Answer from the drawing. Dimensions are ordinates in mm from the lowest x, y and z of the part. A direction names the side the tool comes from. Give positions to 0.01 mm unless a question says otherwise; leave off trailing zeros. Loops run counter-clockwise (first coordinate to the right, second up) from the corner with the lowest first, then second, coordinate; pieces in that order, holes last.
Item 1: Consider line 1 along X through (y, z) = (29, 45) (1 decimal); line 2 along Y through (x, z) = (159, 42); line 3 along Z through (x, y) = (75.5, 66.5). Determine where each line is inside the solid, lowest interval first.
Item 2: Section B-B, the plane y = 73.5 is taken. Give the vertices of the cut face in (x, z) (1 decimal), and give its area (3 significant figures).
Item 3: Each of these flat-tipped pins is pushed along its axis until it touches: pin 1 Ø6 at (x, y) = (158, 87) entering from -Z; pin 2 Ø5 at (x, y) = (4, 69) entering from +Z; pin 3 Ø7.5 at (x, y) = (71.5, 105.5) entering from +Z; pin 4 Ø6 at (x, y) = (191, 23) entering from +Z. Where does it stop, or does it pass through?
Item 4: Section C-C, the plane z = 44 is taken. Give the vertices of the cut face in (x, y) (1 decimal), and give its area (3 significant figures).
Item 5: The mould has two halves that part along X. Classify the marked faces 3, 4 and 5: pulls with the +X half, pulls with the -X half, needs draft (parallel to the pull), parting line crosses it, or undercut.
Item 6: Section A-A, the plane x = 41 is taken. Give the vertices of the cut face in (y, z), and give its area (3 significant figures).
Item 7: A tool of negligible diameter and unlimited length cuts with its end or side. For the marked faces 1 and 2, from which of +Z, -Z, +X, -X, +Y, -Y can it reach the whole face along a straight path? Write none if from no direction.
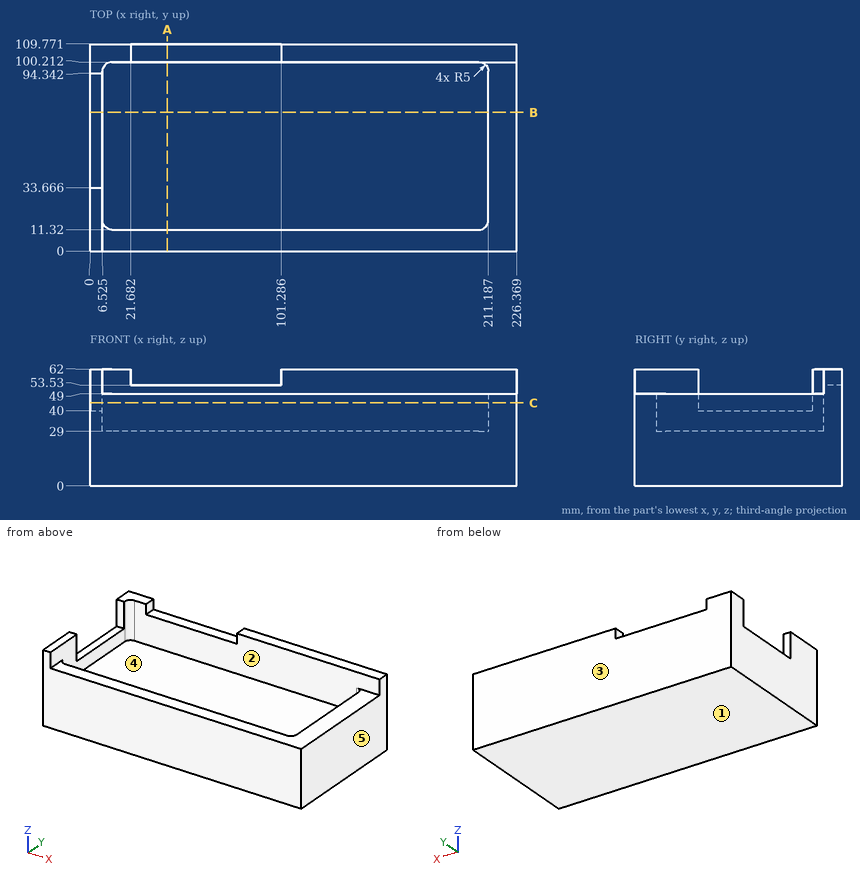
Worked answers:
1. line 1: x = 0 to 6.5, 211.2 to 226.4
1. line 2: y = 0 to 11.32, 100.21 to 109.77
1. line 3: z = 0 to 29
2. outline: (0, 0) - (226.4, 0) - (226.4, 49) - (211.2, 49) - (211.2, 29) - (6.5, 29) - (6.5, 40) - (0, 40) - close
2. area: 6,940 mm2
3. pin 1: stops at z = 0
3. pin 2: stops at z = 40
3. pin 3: stops at z = 53.53
3. pin 4: stops at z = 29
4. outline: (0, 0) - (226.4, 0) - (226.4, 109.8) - (0, 109.8) - (0, 94.3) - (6.5, 94.3) - (6.5, 95.2) arc R5 cw to (11.5, 100.2) - (206.2, 100.2) arc R5 cw to (211.2, 95.2) - (211.2, 16.3) arc R5 cw to (206.2, 11.3) - (11.5, 11.3) arc R5 cw to (6.5, 16.3) - (6.5, 33.7) - (0, 33.7) - close
4. area: 6,280 mm2
5. face 3: needs draft
5. face 4: undercut
5. face 5: pulls with the +X half
6. outline: (0, 0) - (109.77, 0) - (109.77, 53.53) - (100.21, 53.53) - (100.21, 29) - (11.32, 29) - (11.32, 49) - (0, 49) - close
6. area: 3,640 mm2
7. face 1: -Z, +X, -X, +Y, -Y
7. face 2: +Z
